Autodesk Inventor part; units mm, degrees
ref_plane "YZ Plane" through (0, 0, 0) normal (1, 0, 0) x (0, 1, 0)
ref_plane "XZ Plane" through (0, 0, 0) normal (0, 1, 0) x (-1, 0, 0)
ref_plane "XY Plane" through (0, 0, 0) normal (0, 0, 1) x (1, 0, 0)
sketch "草圖1" plane through (0, 0, 0) normal (0, 1, 0) x (-1, 0, 0)
  circle A0 centre (0, 0) radius 4
  circle A1 centre (0, 0) radius 12.5
  dimension "d0" = 8
  dimension "d1" = 25
extrude "擠出1" add sketch "草圖1" along normal blind 13
sketch "草圖2" plane through (0, 13, 0) normal (0, 1, 0) x (1, 0, 0)
  circle A0 centre (0, 0) radius 19.5
  circle A1 centre (0, 0) radius 4
  dimension "d4" = 39
extrude "擠出2" add sketch "草圖2" along normal blind 5
sketch "草圖3" plane through (0, 18, 0) normal (0, 1, 0) x (1, 0, 0)
  circle A0 centre (0, 0) radius 16 construction
  circle A1 centre (-16, 0) radius 1.75
  circle A2 centre (0, -16) radius 1.75
  circle A3 centre (16, 0) radius 1.75
  circle A4 centre (0, 16) radius 1.75
  dimension "d7" = 32
  dimension "d8" = 3.5
  dimension "d11" = 360
extrude "擠出3" cut sketch "草圖3" against normal blind 5
properties part number "8 mm hub"
Geometry: final body of the model. Coordinates: model frame, mm. A direction names the side the tool comes from. Give positions to 0.01 mm unless a question says otherwise; leave off trailing zeros. Write each loop counter-clockwise with the first axis right and the second up, starting at its lowest first coordinate (ties: lowest second). Pieces come first, ordered by that corner, then holes.
1. Section query C-C, the plane y = 14.5. Return loops of the section in (x, z), then the cut area to 3 significant figures.
2. Line query: probe 1 along Z at (x, y) = (0, 16.5); probe 2 along Z at (x, y) = (0, 9). Output: solid intervals per line, ascending.
3. Pin query (flat end, axial travel): P1, Ø2, axis at x = 16, z = 0, coming from the -Y side; P2, Ø5.5, axis at x = -16, z = 0, coming from the -Y side; P3, Ø10, axis at x = -5.5, y = 16, coming from the -Z side; P4, Ø3, axis at y = 12.5, z = -14.5, coming from the -X side. Return the tip coordinate at first contact, or that it passes through.
4. Reachability of faces 1 (the flat face through (0, 13, 13)), 2 (the flat face through (0, 18, -5)) from +Z, -Z, +X, -X, +Y, -Y: full face, straight path, thin tool, end or side. Return the list, or none.
5. Section query D-D, the plane z = -16. Return loops of the section in (x, y).
6. Section query B-B, the plane z = 7.5. Return loops of the section in (x, y), then the cut area to 3 significant figures.
Computed:
1. outline: circle Ø39 at (0, 0); hole circle Ø3.5 at (-16, 0); hole circle Ø8 at (0, 0); hole circle Ø3.5 at (0, -16); hole circle Ø3.5 at (0, 16); hole circle Ø3.5 at (16, 0)
1. area: 1,110 mm2
2. probe 1: z = -19.5 to -17.75, -14.25 to -4, 4 to 14.25, 17.75 to 19.5
2. probe 2: z = -12.5 to -4, 4 to 12.5
3. P1: passes through
3. P2: stops at y = 13
3. P3: stops at z = -19.49
3. P4: stops at x = -14.46
4. face 1: -Y
4. face 2: +Z, -Z, +X, -X, +Y
5. outline: (-11.15, 13) - (-1.75, 13) - (-1.75, 18) - (-11.15, 18) - close; (1.75, 13) - (11.15, 13) - (11.15, 18) - (1.75, 18) - close
6. outline: (-18, 13) - (-10, 13) - (-10, 0) - (10, 0) - (10, 13) - (18, 13) - (18, 18) - (-18, 18) - close
6. area: 440 mm2
